Work out the finished part from the listing and answer in its coordinate system (mm). Face numbers are marked on the shaded views. A direction names the side the tool comes from. Round coordinates to 2 decimals unless told otherwise and drop trailing zeros. Order: outer loops, then holes, each group sorted by start corner. A loop starts at its lowest first (then second) coordinate and runs counter-clockwise, first axis right, second up. Notation, with made-up numbers: (6.25, 23.25) - (30.25, 23.25) arc R8 cw to (30.25, 34.25) - close; hole circle Ø3 at (-2.5, 70.5). An arc over 180 degrees is marked (long way). Put each result on its own line as item: value.
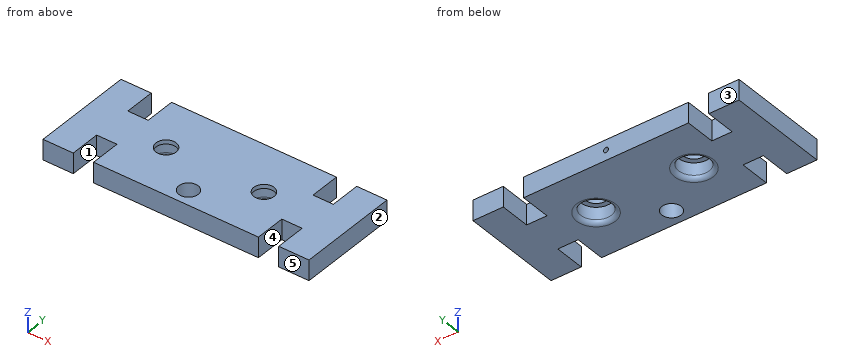
Autodesk Inventor part; units mm, degrees
ref_plane "Work Plane1" through (-40.6, 25, 0) normal (0, 1, 0) x (1, 0, 0)
ref_plane "YZ Plane" through (0, 0, 0) normal (1, 0, 0) x (0, 1, 0)
ref_plane "XZ Plane" through (0, 0, 0) normal (0, 1, 0) x (-1, 0, 0)
sketch "Sketch1" plane through (0, 0, 0) normal (0, 0, 1) x (1, 0, 0)
  line L0 (65.5, 25) -> (-65.5, 25)
  line L1 (-65.5, 25) -> (-65.5, -25)
  line L2 (-65.5, -25) -> (65.5, -25)
  line L3 (65.5, -25) -> (65.5, 25)
  line L4 (-40.6, 25) -> (-40.6, 10)
  line L5 (-40.6, 10) -> (-50.6, 10)
  line L6 (-50.6, 10) -> (-50.6, 25)
  line L7 (-40.6, -25) -> (-40.6, -10)
  line L8 (-40.6, -10) -> (-50.6, -10)
  line L9 (-50.6, -10) -> (-50.6, -25)
  line L10 (40.6, 25) -> (40.6, 10)
  line L11 (40.6, 10) -> (50.6, 10)
  line L12 (50.6, 10) -> (50.6, 25)
  line L13 (40.6, -25) -> (40.6, -10)
  line L14 (40.6, -10) -> (50.6, -10)
  line L15 (50.6, -10) -> (50.6, -25)
  circle A0 centre (24.1, 0) radius 7.5
  circle A1 centre (-24.1, 0) radius 7.5
  line L16 (0, -25) -> (0, -17)
  circle A2 centre (0, -17) radius 4.75
  circle A3 centre (-24.1, 0) radius 5
  circle A4 centre (24.1, 0) radius 5
  point P0 (0, 0)
  point P1 (0, 0)
  dimension "d0" = 15
  dimension "d1" = 15
  dimension "d2" = 15
  dimension "d3" = 15
  dimension "d8" = 15
  dimension "d9" = 15
  dimension "d23" = 8
  dimension "d24" = 9.5
  dimension "d27" = 10
  dimension "d28" = 10
ref_plane "Work Plane1" through (-40.6, 25, 0) normal (0, 1, 0) x (1, 0, 0)
sketch "Sketch2" plane through (-40.6, 25, 0) normal (0, 1, 0) x (1, 0, 0)
  circle A0 centre (40.6, -5) radius 1.25
  point P0 (40.6, 0)
  dimension "d20" = 2.5
extrude "Extrusion11" add sketch "Sketch1" along normal blind 10 contours L3 L2 L15 L14 L13 L7 L8 L9 L1 L0 L6 L5 L4 L10 L11 L12 | A0 | A1
extrude "Extrusion12" cut sketch "Sketch1" along normal blind 8 contours A0 | A1
sketch "Sketch4" plane through (-40.6, 25, 0) normal (0, 1, 0) x (1, 0, 0)
  line L0 (40.6, 0) -> (40.6, -5)
  circle A0 centre (40.6, -5) radius 1.25
  dimension "d50" = 5
  dimension "d51" = 2.5
extrude "Extrusion14" cut sketch "Sketch4" against normal blind 10
fillet "Fillet1" radius 2 2 edges at (-31.6, 0, 0) (16.6, 0, 0)
properties part number "prepazka_2x_lozisko_1x_dira"
1) Straight lines are drawn through the part: L1, parallel to X at y = -17, z = 7.75; L2, parallel to X at y = -22.5, z = 6.5; L3, parallel to X at y = 22, z = 5.25. For each, find the intervals that lie inside material, in ascending order. Write a range as from..to.
Findings below:
L1: x = -65.5..-50.6, -40.6..-4.75, 4.75..40.6, 50.6..65.5
L2: x = -65.5..-50.6, -40.6..40.6, 50.6..65.5
L3: x = -65.5..-50.6, -40.6..-1.22, 1.22..40.6, 50.6..65.5
2) A cutting plane is placed at B-B on y = -17. Write down the section's boundary in (x, z).
Findings below:
outline: (-65.5, 0) - (-50.6, 0) - (-50.6, 10) - (-65.5, 10) - close; (-40.6, 0) - (-4.75, 0) - (-4.75, 10) - (-40.6, 10) - close; (4.75, 0) - (40.6, 0) - (40.6, 10) - (4.75, 10) - close; (50.6, 0) - (65.5, 0) - (65.5, 10) - (50.6, 10) - close
3) A cutting plane is placed at D-D on x = 0. Write down the section's boundary in (y, z).
Findings below:
outline: (-25, 0) - (-21.75, 0) - (-21.75, 10) - (-25, 10) - close; (-12.25, 0) - (25, 0) - (25, 3.75) - (15, 3.75) - (15, 6.25) - (25, 6.25) - (25, 10) - (-12.25, 10) - close
4) Given pin 1 Ø6 at (x, z) = (-41, 5) entering from -Y; pin 2 Ø9 at (x, y) = (24.1, 0) entering from -Z; pin 3 Ø13.5 at (x, y) = (-24.1, 0) entering from -Z; pin 4 Ø0.8 at (x, z) = (0.5, 5) entering from +Y, each flat-ended and moving along its own axis, determine where each tip first touches the part or whether it passes through.
Findings below:
pin 1: stops at y = -25
pin 2: passes through
pin 3: stops at z = 8
pin 4: stops at y = 15
5) A cutting plane is placed at A-A on x = 24.1. Write down the section's boundary in (y, z), then the cut area to 3 significant figures.
Findings below:
outline: (-25, 0) - (-9.5, 0) arc R2 ccw to (-7.5, 2) - (-7.5, 8) - (-5, 8) - (-5, 10) - (-25, 10) - close; (5, 8) - (7.5, 8) - (7.5, 2) arc R2 ccw to (9.5, 0) - (25, 0) - (25, 10) - (5, 10) - close
area: 358 mm2
6) For the marked faces 4 and 5, determine the directions among +Z, -Z, +X, -X, +Y, -Y from which every point of the face is accessible in a straight line to the end or side of a thin tool.
Findings below:
face 4: +Z, -Z, -Y
face 5: +Z, -Z, +X, -X, -Y
7) A cutting plane is placed at C-C on y = 0. Write down the section's boundary in (x, z).
Findings below:
outline: (-65.5, 0) - (-33.6, 0) arc R2 ccw to (-31.6, 2) - (-31.6, 8) - (-29.1, 8) - (-29.1, 10) - (-65.5, 10) - close; (-19.1, 8) - (-16.6, 8) - (-16.6, 2) arc R2 ccw to (-14.6, 0) - (14.6, 0) arc R2 ccw to (16.6, 2) - (16.6, 8) - (19.1, 8) - (19.1, 10) - (-19.1, 10) - close; (29.1, 8) - (31.6, 8) - (31.6, 2) arc R2 ccw to (33.6, 0) - (65.5, 0) - (65.5, 10) - (29.1, 10) - close
8) For a pull along X with two mould halves and no side action, classify the marked faces 1, 2 and 3 as pulls with the +X half, pulls with the -X half, needs draft (parallel to the pull), parting line crosses it, or undercut.
Findings below:
face 1: undercut
face 2: pulls with the +X half
face 3: needs draft
